Check sheet for the modelled part. Datum: model origin and axes. Units: mm. A direction names the side the tool comes from. Give positions to 0.01 mm unless a question says otherwise; leave off trailing zeros. Loops run counter-clockwise (first coordinate to the right, second up) from the corner with the lowest first, then second, coordinate; pieces in that order, holes last. Notation, with made-up numbers: (20.25, 55) - (40.25, 55) arc R20 ccw to (40.25, 64) - close; hole circle Ø8 at (19, -8). An arc over 180 degrees is marked (long way). Answer in a Markdown table with one row per item. Add a question column.
(1) Draft check along Z on faces 4 (the face through (-2, 23, 149.5)), 5 (the face through (144, 35, -142.5)), 6 (the face through (2, 4, 2)), 7 (the face through (162, 54, 2)). Enter one of: released by +Z, released by -Z, zero draft, split by the parting line, or undercut.
(2) Thickness scan on L1, parallel to X at y = 19, z = 120.5; L2, parallel to Z at x = -66.5, y = 32.5; L3, parallel to Y at x = 26.5, z = -72. Record the ranges inside material, lowest first.
(3) Sectioned sample at C-C on x = 40. Enter the section's corners in (y, z), then the cut area to 3 significant figures.
(4) Sectioned sample at A-A on y = 19. Enter the section's corners in (x, z).
(5) Go/stop test with flat-tipped pins: P1, Ø6, axis at y = 31.5, z = -105, coming from the +X side; P2, Ø12, axis at y = 35.5, z = 17.5, coming from the -X side; P3, Ø8, axis at x = 48.5, z = -50, coming from the +Y side; P4, Ø11, axis at x = -154, y = 24.5, coming from the -Z side. Record where each tip stops, or that it passes through.
(6) Set-up check for faces 1 (the face through (-138, 20, 148)), 2 (the face through (138, 20, -148)), 3 (the face through (-162, 50, 2)): record each of +Z, -Z, +X, -X, +Y, -Y from which the full face is reachable in a straight line by a thin tool's end or side.
(7) Sectioned sample at B-B on z = 106. Enter the section's corners in (x, y).
from build123d import *

# Parameters (mm, degrees)
BASE_FLANGIA1_DEPTH       = 142.5
BORDO_FLANGIA1_DEPTH      = 276
BORDO_FLANGIA1_BEND_DEPTH = 276


# Sheet-metal steps are written as plain solids
with BuildPart() as part:
    # Schizzo1 → Base-Flangia1 (new, symmetric)
    with BuildSketch(Plane.XY):
        with BuildLine():
            Line((-175, 50), (-148, 50))
            ThreePointArc((-148, 50), (-145.878679656, 49.121320344), (-145, 47))
            Line((-145, 47), (-145, 7))
            ThreePointArc((-145, 7), (-142.949747468, 2.050252532), (-138, 0))
            Line((-138, 0), (138, 0))
            ThreePointArc((138, 0), (142.949747468, 2.050252532), (145, 7))
            Line((145, 7), (145, 47))
            ThreePointArc((145, 47), (145.878679656, 49.121320344), (148, 50))
            Line((148, 50), (175, 50))
            Line((175, 50), (175, 54))
            Line((175, 54), (148, 54))
            ThreePointArc((148, 54), (143.050252532, 51.949747468), (141, 47))
            Line((141, 47), (141, 7))
            ThreePointArc((141, 7), (140.121320344, 4.878679656), (138, 4))
            Line((138, 4), (-138, 4))
            ThreePointArc((-138, 4), (-140.121320344, 4.878679656), (-141, 7))
            Line((-141, 7), (-141, 47))
            ThreePointArc((-141, 47), (-143.050252532, 51.949747468), (-148, 54))
            Line((-148, 54), (-175, 54))
            Line((-175, 54), (-175, 50))
        make_face()
    extrude(amount=BASE_FLANGIA1_DEPTH, both=True)

    # Bordo-Flangia1 section (across the edge) → Bordo-Flangia1 (add)
    with BuildSketch(Plane(origin=(-138, 4, 145.5), x_dir=(0, 0, -1), z_dir=(1, 0, 0))):
        with BuildLine():
            Line((-4, 3), (-4, 36))
            Line((-4, 36), (0, 36))
            Line((0, 36), (0, 3))
            ThreePointArc((0, 3), (0.878679656, 0.878679656), (3, 0))
            Line((3, 0), (3, -4))
            ThreePointArc((3, -4), (-1.949747468, -1.949747468), (-4, 3))
        make_face()
    extrude(amount=BORDO_FLANGIA1_DEPTH)

    # Bordo-Flangia1 section 2 (across the edge) → Bordo-Flangia1 bend (add)
    with BuildSketch(Plane(origin=(138, 4, -145.5), x_dir=(0, 0, 1), z_dir=(-1, 0, 0))):
        with BuildLine():
            Line((-4, 3), (-4, 36))
            Line((-4, 36), (0, 36))
            Line((0, 36), (0, 3))
            ThreePointArc((0, 3), (0.878679656, 0.878679656), (3, 0))
            Line((3, 0), (3, -4))
            ThreePointArc((3, -4), (-1.949747468, -1.949747468), (-4, 3))
        make_face()
    extrude(amount=BORDO_FLANGIA1_BEND_DEPTH)


solid = part.part
Reply:
| question | item | result |
|---|---|---|
| 1 | face 4 | released by +Z |
| 1 | face 5 | released by -Z |
| 1 | face 6 | undercut |
| 1 | face 7 | zero draft |
| 2 | L1 | -145 to -141, 141 to 145 |
| 2 | L2 | -149.5 to -145.5, 145.5 to 149.5 |
| 2 | L3 | 0 to 4 |
| 3 | outline | (0, -142.5) arc R7 ccw to (7, -149.5) - (40, -149.5) - (40, -145.5) - (7, -145.5) arc R3 cw to (4, -142.5) - (4, 142.5) arc R3 cw to (7, 145.5) - (40, 145.5) - (40, 149.5) - (7, 149.5) arc R7 ccw to (0, 142.5) - close |
| 3 | area | 1,470 mm^2 |
| 4 | outline | (-145, -142.5) - (-141, -142.5) - (-141, 142.5) - (-145, 142.5) - close; (-138, -149.5) - (138, -149.5) - (138, -145.5) - (-138, -145.5) - close; (-138, 145.5) - (138, 145.5) - (138, 149.5) - (-138, 149.5) - close; (141, -142.5) - (145, -142.5) - (145, 142.5) - (141, 142.5) - close |
| 5 | P1 | x = 145 |
| 5 | P2 | x = -145 |
| 5 | P3 | y = 4 |
| 5 | P4 | through |
| 6 | face 1 | +Z, -X, +Y, -Y |
| 6 | face 2 | -Z, +X, +Y, -Y |
| 6 | face 3 | +Z, -Z, -X, -Y |
| 7 | outline | (-175, 50) - (-148, 50) arc R3 cw to (-145, 47) - (-145, 7) arc R7 ccw to (-138, 0) - (138, 0) arc R7 ccw to (145, 7) - (145, 47) arc R3 cw to (148, 50) - (175, 50) - (175, 54) - (148, 54) arc R7 ccw to (141, 47) - (141, 7) arc R3 cw to (138, 4) - (-138, 4) arc R3 cw to (-141, 7) - (-141, 47) arc R7 ccw to (-148, 54) - (-175, 54) - close |
